The listing builds one solid part. Answer for the finished solid, in the listing's coordinates (mm). A direction names the side the tool comes from. Give positions to 0.01 mm unless a question says otherwise; leave off trailing zeros. Write each loop counter-clockwise with the first axis right and the second up, starting at its lowest first coordinate (ties: lowest second). Pieces come first, ordered by that corner, then holes. Notation, with made-up numbers: (48.25, 51.25) - (91.25, 51.25) arc R17 cw to (91.25, 68.25) - close; hole circle Ø7 at (-21, 41.25). An arc over 180 degrees is marked (long way). Return JSON: item names as keys, results as strings.
from build123d import *

# Parameters (mm, degrees)
F1_DEPTH = 10
F2_W     = 30
F2_H     = 20
F3_DEPTH = 20
F4_SIZE2 = 9.99999
F4_SIZE  = 19.99999


# Not quite as in the source:
# - a fillet or chamfer is up to 0.001 mm smaller than in the source, because OpenCascade refuses the exact size


with BuildPart() as f1:
    # F0 (on Top) → F1 (new body)
    with BuildSketch(Plane.XY):
        Polygon((0, 30), (0, 0), (20, 0), (20, -10), (30, -10), (60, 30), align=None)
    extrude(amount=F1_DEPTH)

    # F2 (on face) → F3 (join)
    with BuildSketch(Plane.XY.offset(10)):
        with Locations((15, 20)):
            Rectangle(F2_W, F2_H)
    extrude(amount=F3_DEPTH)

    # F4 (size 20 and 10 in the source; OpenCascade refuses exactly that, so slightly less here)
    f4_edges = [f1.edges().sort_by_distance(p)[0] for p in [
        (15, 10, 30),
    ]]
    f4_side = f1.faces().sort_by_distance((15, 20, 30))[0]
    chamfer(f4_edges, length=F4_SIZE, length2=F4_SIZE2, reference=f4_side)


solid = f1.part
Item 1: For faces 1 (the face through (30, 20, 18)), 2 (the face through (23, 15, 0)), 3 (the face through (20, -5, 5)), 4 (the face through (15, 10, 15)), 5 (the face through (0, 18, 11)), determine the directions among +Z, -Z, +X, -X, +Y, -Y from which every point of the face is accessible in a straight line to the end or side of a thin tool.
Answer below:
{"face 1": "+Z, +X, +Y, -Y", "face 2": "-Z, +X, -X, +Y, -Y", "face 3": "+Z, -Z, -X, -Y", "face 4": "+Z, +X, -X, -Y", "face 5": "+Z, -Z, -X, +Y, -Y"}
Item 2: A cutting plane is placed at C-C on z = 4.75. Determine the outline of the cut face in (x, y), then the cut area to 3 significant figures.
Answer below:
{"outline": "(0, 0) - (20, 0) - (20, -10) - (30, -10) - (60, 30) - (0, 30) - close", "area": "1,600 mm²"}
Item 3: A cutting plane is placed at B-B on y = 24. Determine the outline of the cut face in (x, z), then the cut area to 4 significant figures.
Answer below:
{"outline": "(0, 0) - (55.5, 0) - (55.5, 10) - (30, 10) - (30, 27) - (0, 27) - close", "area": "1,065 mm²"}
Item 4: Flat-ended cylindrical pins translate along their axes: P1, Ø5, axis at x = 22.5, z = 13.5, coming from the -Y side; P2, Ø3, axis at x = 50, y = 26, coming from the +Z side; P3, Ø8, axis at x = 8, z = 5.5, coming from the -Y side. Find the tip coordinate at first contact, or state that the pin passes through.
Answer below:
{"P1": "stops at y = 10", "P2": "stops at z = 10", "P3": "stops at y = 0"}
Item 5: Consider L1, parallel to Y at x = 13, z = 19.75; L2, parallel to X at y = 28, z = 20; L3, parallel to Z at x = 43.5, y = 12.5. Determine where each line is inside the solid, lowest interval first.
Answer below:
{"L1": "y = 10 to 30", "L2": "x = 0 to 30", "L3": "z = 0 to 10"}
